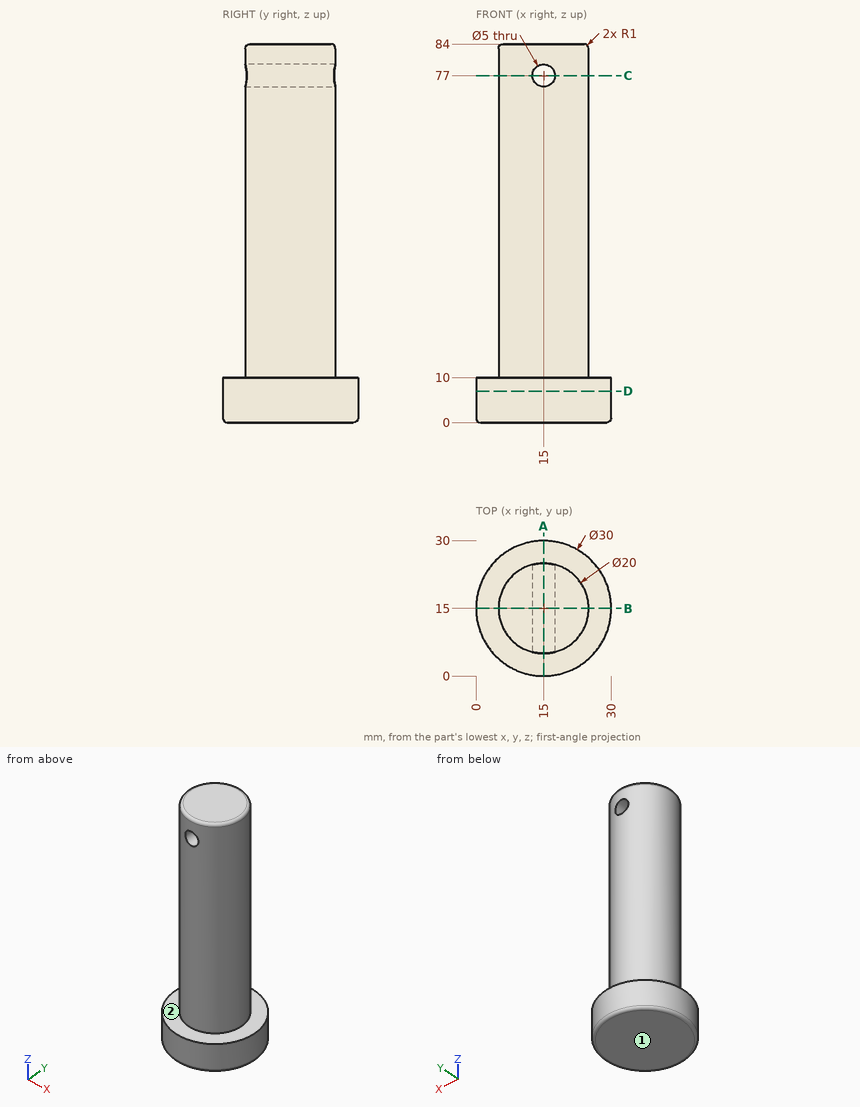
Answer from the drawing. Dimensions are ordinates in mm from the lowest x, y and z of the part. A direction names the side the tool comes from. Coordinates: 2 decimals unless noted, no trailing zeros. Write each loop counter-clockwise with the first axis right and the second up, starting at its lowest first coordinate (ties: lowest second). Pieces come first, ordered by that corner, then holes. Notation, with made-up numbers: M 67,-31 L 113,-31 A20 ccw 113,-15 Z; hole C 12.25,21 d10. An arc over 180 degrees is marked long. Write item = value, one per line.
1. Flat-ended cylindrical pins translate along their axes: pin 1 (1.5 mm diameter, centred on y = 23.5, z = 60, fed in from -X); pin 2 (8 mm diameter, centred on x = 6, z = 56.5, fed in from +Y); pin 3 (12 mm diameter, centred on x = 4.5, z = 71.5, fed in from -Y). Find the tip coordinate at first contact, or state that the pin passes through.
Solution:
pin_1 = 8.68
pin_2 = 23.66
pin_3 = 6.07
2. For the marked faces 1 and 2, determine the directions among +Z, -Z, +X, -X, +Y, -Y from which every point of the face is accessible in a straight line to the end or side of a thin tool.
Solution:
face_1 = -Z, +X, -X, +Y, -Y
face_2 = +Z
3. The part is cut by section B-B (y = 15). Determine the outline of the cut face in (x, z).
Solution:
outline = M 0,1 A1 ccw 1,0 L 29,0 A1 ccw 30,1 L 30,10 L 25,10 L 25,83 A1 ccw 24,84 L 6,84 A1 ccw 5,83 L 5,10 L 0,10 Z; hole C 15,77 d5
4. The part is cut by section D-D (z = 7). Determine the outline of the cut face in (x, y), then the cut area to 3 significant figures.
Solution:
outline = C 15,15 d30
area = 707 mm2
5. Straight lines are drawn through the part: line 1 (Z direction, x = 15, y = 19.75); line 2 (Z direction, x = 4.5, y = 7.75); line 3 (X direction, y = 19, z = 77). For each, find the intervals that lie inside material, in ascending order. Write a range as from..to.
Solution:
line_1 = 0..74.5, 79.5..84
line_2 = 0..10
line_3 = 5.83..12.5, 17.5..24.17
6. The part is cut by section A-A (x = 15). Determine the outline of the cut face in (y, z), then the cut area to 3 significant figures.
Solution:
outline = M 0,1 A1 ccw 1,0 L 29,0 A1 ccw 30,1 L 30,10 L 25,10 L 25,74.5 L 5,74.5 L 5,10 L 0,10 Z; M 5,79.5 L 25,79.5 L 25,83 A1 ccw 24,84 L 6,84 A1 ccw 5,83 Z
area = 1,680 mm2
7. The part is cut by section C-C (z = 77). Determine the outline of the cut face in (x, y).
Solution:
outline = M 12.5,5.32 L 12.5,24.68 A10 ccw Z; M 17.5,5.32 A10 ccw 17.5,24.68 Z
